```python
from build123d import *

# Parameters (mm, degrees)
BOSS_EXTRUDE1_DEPTH = 38.1
SKETCH4_W           = 19.05
SKETCH4_H           = 25.4
CUT_EXTRUDE1_START  = -6.35
CUT_EXTRUDE1_DEPTH  = 6.35
CIRPATTERN1_COUNT   = 13
CIRPATTERN1_ANGLE   = 140
CIRPATTERN2_COUNT   = 4
CIRPATTERN2_ANGLE   = 120
SKETCH13_W          = 4.452036414
SKETCH13_H          = 6.35
CUT_REVOLVE2_ANGLE  = 145
FILLET1_R           = 5.08


with BuildPart() as part:
    # Sketch1 → Boss-Extrude1 (new body)
    with BuildSketch(Plane(origin=(0, 0, 0), x_dir=(1, 0, 0), z_dir=(0, 1, 0))):
        with BuildLine():
            Line((-110.390390627, -40.178816337), (-86.522198059, -31.491504697))
            ThreePointArc((-86.522198059, -31.491504697), (0, -92.075), (86.522198059, -31.491504697))
            Line((86.522198059, -31.491504697), (110.390390627, -40.178816337))
            ThreePointArc((110.390390627, -40.178816337), (0, -117.475), (-110.390390627, -40.178816337))
        make_face()
    extrude(amount=-BOSS_EXTRUDE1_DEPTH)

    # Sketch4 → Cut-Revolve1 (revolve, cut)
    with BuildSketch(Plane(origin=(86.522198059, 0, 31.491504697), x_dir=(0.9396926207859084, 0, 0.34202014332566905), z_dir=(-0.34202014332566905, 0, 0.9396926207859084))):
        with Locations((9.525, -19.05)):
            Rectangle(SKETCH4_W, SKETCH4_H)
    revolve(axis=Axis((0, -38.1, 0), (0, 1, 0)), mode=Mode.SUBTRACT)

    # Sketch5 → Cut-Extrude1 (cut)
    with BuildSketch(Plane(origin=(0, -31.75, 0), x_dir=(1, 0, 0), z_dir=(0, 1, 0)).offset(CUT_EXTRUDE1_START)):
        Polygon((98.301392685, -45.398059752), (88.621295381, -40.60893497), (86.049357998, -45.807505744), (95.729455302, -50.596630526), align=None)
    cut_extrude1 = extrude(amount=CUT_EXTRUDE1_DEPTH, mode=Mode.SUBTRACT)

    # CirPattern1: Cut-Extrude1 ×13 about axis
    cirpattern1_axis = Axis((0, 0, 0), (0, -1, 0))
    for i in range(1, CIRPATTERN1_COUNT):
        add(cut_extrude1.rotate(cirpattern1_axis, i * CIRPATTERN1_ANGLE / (CIRPATTERN1_COUNT - 1)), mode=Mode.SUBTRACT)

    # Sketch11 → #8-32 Tapped Hole1 (revolve, cut)
    with BuildSketch(Plane(origin=(90.737811682, 0, 52.3875), x_dir=(0, 0, 1), z_dir=(1, 0, 0))):
        Polygon((0, 0), (0, 11.705806461), (1.7272, 10.668), (1.7272, 0), align=None)
    f_8_32_tapped_hole1 = revolve(axis=Axis((90.737811682, 6.35, 52.3875), (0, -1, 0)), mode=Mode.SUBTRACT)

    # CirPattern2: #8-32 Tapped Hole1 ×4 about axis
    cirpattern2_axis = Axis((0, 0, 0), (0, -1, 0))
    for i in range(1, CIRPATTERN2_COUNT):
        add(f_8_32_tapped_hole1.rotate(cirpattern2_axis, i * CIRPATTERN2_ANGLE / (CIRPATTERN2_COUNT - 1)), mode=Mode.SUBTRACT)

    # Sketch13 → Cut-Revolve2 (revolve, cut)
    with BuildSketch(Plane(origin=(0, 0, 0), x_dir=(-0.9396926207859083, 0, -0.3420201433256694), z_dir=(0.3420201433256694, 0, -0.9396926207859083))):
        with Locations((-94.301018207, -34.925)):
            Rectangle(SKETCH13_W, SKETCH13_H)
    revolve(axis=Axis((0, -38.1, 0), (0, -1, 0)), revolution_arc=CUT_REVOLVE2_ANGLE, mode=Mode.SUBTRACT)

    # Fillet1
    fillet1_edges = [part.edges().sort_by_distance(p)[0] for p in [
        (-90.705743825, -34.925, 33.014190829),
        (90.705743825, -34.925, 33.014190829),
    ]]
    fillet(fillet1_edges, radius=FILLET1_R)


solid = part.part
```
Work out the finished part from the listing and answer in its coordinate system (mm). A direction names the side the tool comes from. Give positions to 0.01 mm unless a question says otherwise; leave off trailing zeros. Loops run counter-clockwise (first coordinate to the right, second up) from the corner with the lowest first, then second, coordinate; pieces in that order, holes last. Notation, with made-up numbers: (47.25, 65.25) -> (79.25, 65.25) arc R15 cw to (79.25, 89.25) -> close; hole circle Ø5 at (31.5, 63). An arc over 180 degrees is marked (long way). Put each result on its own line as item: value. Start each with the question number.
Item 1: The mould has two halves that part along Y. Classify faces 1 (the face through (9.114, -34.969, 97.012)), 2 (the face through (-1.9, -18.87, 111.11)): released by +Y, released by -Y, zero draft, split by the parting line, or undercut.
Item 2: Which of the six approach directions +Z, -Z, +X, -X, +Y, -Y give full straight-line access (tool end or side, diameter ignored) to faces 3 (the face through (-1.57, -3.13, 92.06)), 4 (the face through (76.82, -34.97, 59.94)), 5 (the face through (1.583, -34.881, 96.514))?
Item 3: The part is cut by section B-B (y = -16.5). Give the vertices of the cut face in (x, z) (3 decimals), then the cut area to 3 significant figures.
Item 4: Each of these flat-tipped pins is pushed along its axis until it touches: P1, Ø6, axis at y = -10, z = 108.5, coming from the -X side; P2, Ø3, axis at x = 34, y = -5.5, coming from the -Z side; P3, Ø5, axis at y = -10.5, z = 83.5, coming from the -X side. Where does it stop, or does it pass through?
Item 5: The part is cut by section C-C (x = -21). Give the vertices of the cut face in (y, z), then the cut area to 3 significant figures.
Item 6: The part is cut by section A-A (x = 70). Give the vertices of the cut face in (y, z).
Item 7: Find the intervals of material crossed by L1, parallel to Y at x = 74, z = 67; L2, parallel to X at y = -14.5, z = 72.5, in increasing order. Write a range as [from, to].
Answers below:
1. face 1: zero draft
1. face 2: undercut
2. face 3: -Z, +Y, -Y
2. face 4: -Y
2. face 5: -Z, -Y
3. outline: (-110.39, 40.179) -> (-104.423, 38.007) arc R111.125 cw to (104.423, 38.007) -> (110.39, 40.179) arc R117.475 ccw to start
3. area: 1,770 mm2
4. P1: x = -51.67
4. P2: z = 84.96
4. P3: x = -85.08
5. outline: (-38.1, 94.22) -> (-31.75, 94.22) -> (-31.75, 109.12) -> (-6.35, 109.12) -> (-6.35, 89.65) -> (0, 89.65) -> (0, 115.58) -> (-38.1, 115.58) -> close
5. area: 464 mm2
6. outline: (-38.1, 66.46) -> (-31.75, 66.46) -> (-31.75, 77.94) -> (-38.1, 77.94) -> close; (-38.1, 82.56) -> (-31.75, 82.56) -> (-31.75, 86.31) -> (-6.35, 86.31) -> (-6.35, 59.81) -> (0, 59.81) -> (0, 94.34) -> (-38.1, 94.34) -> close
7. L1: [-38.1, -31.75], [-6.35, 0]
7. L2: [-92.43, -84.22], [84.22, 92.43]
